Check sheet for the drawn part. Datum: minimum x, y, z corner. Units: mm. A direction names the side the tool comes from. Coordinates: 2 decimals unless noted, no trailing zeros. Write each loop counter-clockwise with the first axis right and the second up, starting at its lowest first coordinate (ties: lowest second). Pieces come first, ordered by that corner, then holes. Notation, with made-up numbers: M 61.5,84.25 L 74.5,84.25 A29 ccw 74.5,107.25 Z; hole C 78.5,62 d4. An arc over 180 degrees is marked long. Answer in a Markdown table with one row per item.
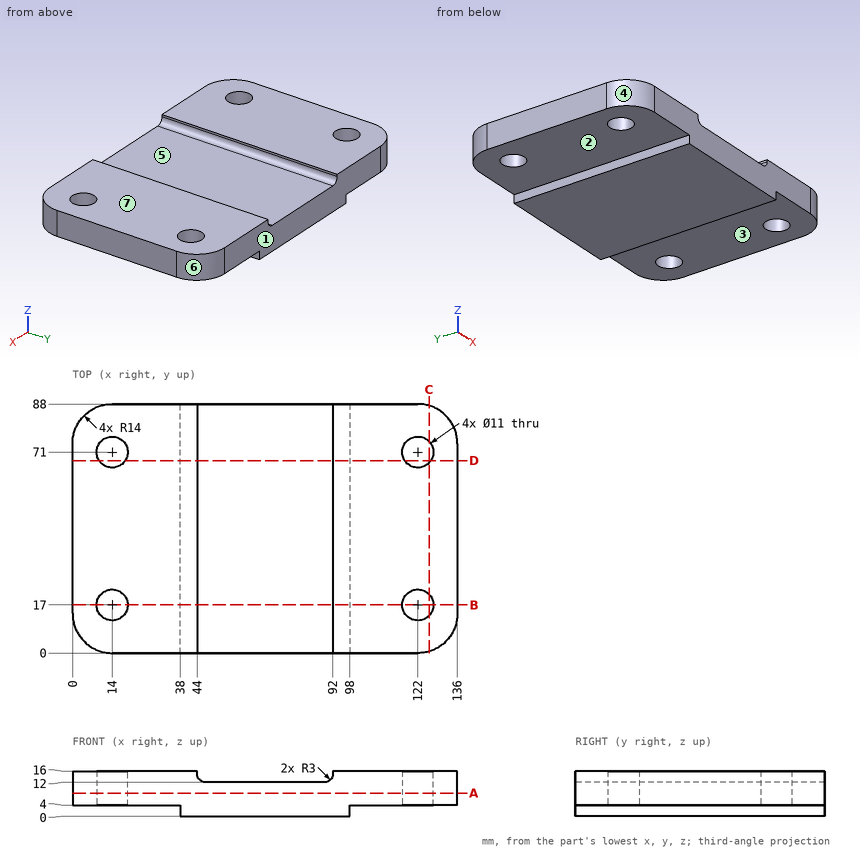
1) Tool access check on the marked faces 1, 2 and 3. Record the directions out of +Z, -Z, +X, -X, +Y, -Y that give a thin tool (end or side, any length) a straight path to the whole face; none if there is none.
Response values:
| item | result |
|---|---|
| face 1 | +Z, -Z, +X, -X, +Y |
| face 2 | -Z, -X, +Y, -Y |
| face 3 | -Z, +X, +Y, -Y |
2) Depth check by flat-ended pin: pin 1 (17.5 mm diameter, centred on x = 122, y = 71, fed in from -Z); pin 2 (3 mm diameter, centred on y = 9, z = 13.5, fed in from -X). Enter the tip coordinate at first touch or a pass-through.
Response values:
| item | result |
|---|---|
| pin 1 | stops at z = 4 |
| pin 2 | stops at x = 0.44 |
3) Thickness scan on L1, parallel to Y at x = 122, z = 10.5; L2, parallel to X at y = 17, z = 7.25; L3, parallel to X at y = 71, z = 12.5. Record the ranges inside material, lowest first. Write a range as [from, to].
Response values:
| item | result |
|---|---|
| L1 | y = [0, 11.5], [22.5, 65.5], [76.5, 88] |
| L2 | x = [0, 8.5], [19.5, 116.5], [127.5, 136] |
| L3 | x = [0, 8.5], [19.5, 45.34], [90.66, 116.5], [127.5, 136] |
4) Sectioned sample at C-C (x = 126). Record the cut outline in (y, z).
Response values:
| item | result |
|---|---|
| outline | M 0.58,4 L 13.23,4 L 13.23,16 L 0.58,16 Z; M 20.77,4 L 67.23,4 L 67.23,16 L 20.77,16 Z; M 74.77,4 L 87.42,4 L 87.42,16 L 74.77,16 Z |
5) Sectioned sample at B-B (y = 17). Record the cut outline in (x, z).
Response values:
| item | result |
|---|---|
| outline | M 0,4 L 8.5,4 L 8.5,16 L 0,16 Z; M 19.5,4 L 38,4 L 38,0 L 98,0 L 98,4 L 116.5,4 L 116.5,16 L 92,16 L 92,15 A3 cw 89,12 L 47,12 A3 cw 44,15 L 44,16 L 19.5,16 Z; M 127.5,4 L 136,4 L 136,16 L 127.5,16 Z |
6) Sectioned sample at A-A (z = 8.25). Record the cut outline in (x, y), then the cut area to 3 significant figures.
Response values:
| item | result |
|---|---|
| outline | M 0,14 A14 ccw 14,0 L 122,0 A14 ccw 136,14 L 136,74 A14 ccw 122,88 L 14,88 A14 ccw 0,74 Z; hole C 14,17 d11; hole C 14,71 d11; hole C 122,17 d11; hole C 122,71 d11 |
| area | 11,400 mm² |
7) Sectioned sample at D-D (y = 68). Record the cut outline in (x, z), then the cut area to 3 significant figures.
Response values:
| item | result |
|---|---|
| outline | M 0,4 L 9.39,4 L 9.39,16 L 0,16 Z; M 18.61,4 L 38,4 L 38,0 L 98,0 L 98,4 L 117.39,4 L 117.39,16 L 92,16 L 92,15 A3 cw 89,12 L 47,12 A3 cw 44,15 L 44,16 L 18.61,16 Z; M 126.61,4 L 136,4 L 136,16 L 126.61,16 Z |
| area | 1,460 mm² |
8) Release check for a two-part mould opening along X. For the marked faces 4, 5, 6 and 7 record: +X half, -X half, draft (parallel to the pull), parting line (faces both ways), or undercut.
Response values:
| item | result |
|---|---|
| face 4 | -X half |
| face 5 | undercut |
| face 6 | +X half |
| face 7 | draft |
